Verification items for the finished model (mm, model axes). Face numbers are marked on the shaded views. A direction names the side the tool comes from. Coordinates: 2 decimals unless noted, no trailing zeros. Loops run counter-clockwise (first coordinate to the right, second up) from the corner with the lowest first, then second, coordinate; pieces in that order, holes last.
Q1. Access from +Z, -Z, +X, -X, +Y, -Y to the whole of each face (thin tool, end or side, straight path). Record for the marked faces 1, 2, 3 and 4.
Q2. Sectioned sample at D-D (z = 10). Enter the section's corners in (x, y).
Q3. Mould release check, pull along Z, two halves, no side actions. Record for the marked faces 5, 6 and 7: +Z half, -Z half, draft (parallel to the pull), parting line (faces both ways), or undercut.
Q4. Go/stop test with flat-tipped pins: P1, Ø6, axis at x = 2, y = 0, coming from the +Z side; P2, Ø4, axis at y = 2.5, z = 18.5, coming from the -X side; P3, Ø14, axis at y = -7, z = 25.5, coming from the +X side. Record where each tip stops, or that it passes through.
Q5. Sectioned sample at C-C (y = 0). Enter the section's corners in (x, z).
Q6. Sectioned sample at A-A (y = -30). Enter the section's corners in (x, z), then the cut area to 3 significant figures.
Q7. Sectioned sample at B-B (x = 10). Enter the section's corners in (y, z), then the cut area to 3 significant figures.
Q8. Material ranges on probe 1 along Y at (x, z) = (0, 28); probe 2 along Y at (x, z) = (-6.5, 3); probe 3 along X at (y, z) = (12, 28.75), recorded low to high.
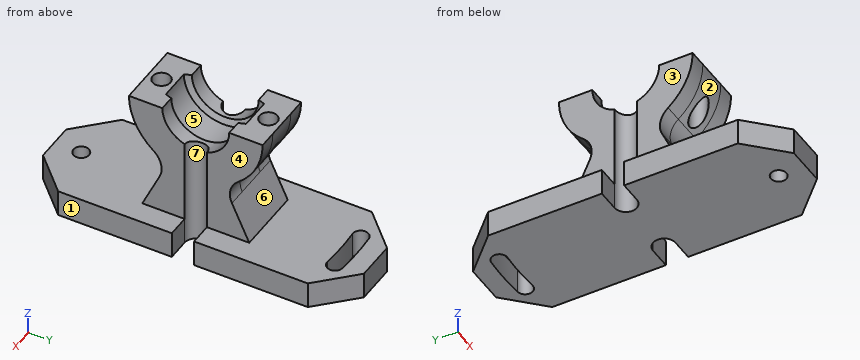
Autodesk Inventor part; units mm, degrees
ref_plane "YZ Plane" through (0, 0, 0) normal (1, 0, 0) x (0, 1, 0)
ref_plane "XZ Plane" through (0, 0, 0) normal (0, 1, 0) x (-1, 0, 0)
ref_plane "XY Plane" through (0, 0, 0) normal (0, 0, 1) x (1, 0, 0)
sketch "Sketch1" plane through (0, 0, 0) normal (1, 0, 0) x (0, 1, 0)
  line L0 (-36, 0) -> (36, 0)
  line L1 (36, 0) -> (36, 6)
  line L2 (36, 6) -> (-36, 6)
  line L3 (-36, 6) -> (-36, 0)
  circle A0 centre (0, 32) radius 9
  circle A1 centre (0, 32) radius 15
  line L4 (0, 32) -> (3.7715, 23.8284) construction
  line L5 (6.2859, 18.3806) -> (12, 6)
  line L6 (0, 32) -> (-3.7715, 23.8284) construction
  line L7 (-6.2859, 18.3806) -> (-12, 6)
  line L8 (15, 32) -> (9, 32)
  line L9 (-9, 32) -> (-15, 32)
  point P0 (0, 0)
  point P1 (0, 0)
  point P2 (12, 32)
  dimension "d3" = 18
  dimension "d4" = 32
  dimension "d5" = 6
  dimension "d6" = 72
  dimension "d7" = 6
  dimension "d44" = 12
  dimension "d45" = 12
extrude "Extrusion1" add sketch "Sketch1" along normal mid plane 7 contours L3 L2 L1 L0 | L7 A1 L5 L2 | A1 L9 A0 L8 picked at (12.871, 30.8714)
sketch "Sketch2" plane through (3.5, 0, 0) normal (1, 0, 0) x (0, 0, -1)
  line L0 (-6, 36) -> (-6, 12)
  line L1 (-6, 12) -> (-18.3806, 6.2859)
  arc A0 (-18.3806, 6.2859) -> (-32, 15) centre (-32, 0) ccw
  line L2 (-32, 15) -> (-32, 9)
  arc A1 (-32, -9) -> (-32, 9) centre (-32, 0) ccw
  line L3 (-32, -9) -> (-32, -15)
  arc A2 (-32, -15) -> (-18.3806, -6.2859) centre (-32, 0) ccw
  line L4 (-18.3806, -6.2859) -> (-6, -12)
  line L5 (-6, -12) -> (-6, -36)
  line L6 (-6, -36) -> (0, -36)
  line L7 (0, -36) -> (0, 36)
  line L8 (0, 36) -> (-6, 36)
  arc A3 (-32, -7.5) -> (-32, 7.5) centre (-32, 0) ccw
  line L9 (-32, 9) -> (-32, 7.5)
  line L10 (-32, -9) -> (-32, -15)
  line L11 (-32, -7.5) -> (-32, -9)
  point P0 (0, 0)
  dimension "d14" = 1.5
extrude "Extrusion2" add sketch "Sketch2" along normal blind 4
sketch "Sketch3" plane through (-3.5, 0, 0) normal (-1, 0, 0) x (0, 0, 1)
  arc A0 (18.3806, -6.2859) -> (32, -15) centre (32, 0) ccw
  line L0 (18.3806, -6.2859) -> (6, -12)
  line L1 (6, -12) -> (6, -36)
  line L2 (6, -36) -> (0, -36)
  line L3 (0, -36) -> (0, 36)
  line L4 (0, 36) -> (6, 36)
  line L5 (6, 36) -> (6, 12)
  line L6 (6, 12) -> (18.3806, 6.2859)
  arc A1 (32, 15) -> (18.3806, 6.2859) centre (32, 0) ccw
  line L7 (32, 15) -> (32, 7.5)
  arc A2 (32, 7.5) -> (32, -7.5) centre (32, 0) ccw
  line L8 (32, -7.5) -> (32, -15)
  point P0 (0, 0)
extrude "Extrusion3" add sketch "Sketch3" along normal blind 4
sketch "Sketch4" plane through (7.5, -36, 0) normal (0, 0, -1) x (-1, 0, 0)
  line L0 (15, 72) -> (15, 0)
  line L1 (0, 0) -> (0, 72)
  line L2 (15, 0) -> (20, 0)
  line L3 (20, 0) -> (20, 72)
  line L4 (20, 72) -> (15, 72)
  line L5 (15, 72) -> (15, 0)
  line L6 (0, 0) -> (-5, 0)
  line L7 (-5, 0) -> (-5, 72)
  line L8 (-5, 72) -> (0, 72)
  line L9 (0, 72) -> (0, 0)
  point P0 (7.5, 36)
  dimension "d17" = 25
extrude "Extrusion4" add sketch "Sketch4" against normal up to surface (6 mm away)
sketch "Sketch5" plane through (3.5, -9, 32) normal (0, 0, 1) x (1, 0, 0)
  line L0 (4, 9) -> (-11, 9)
  line L1 (-11, 9) -> (-31, 9) construction
  line L2 (-11, 1.5) -> (-11, 16.5)
  line L3 (-11, 11.5) -> (-31, 11.5)
  line L4 (-31, 6.5) -> (-11, 6.5)
  arc A0 (-11, 6.5) -> (-11, 11.5) centre (-11, 9) ccw
  arc A1 (-31, 11.5) -> (-31, 6.5) centre (-31, 9) ccw
  line L5 (4, 9) -> (24, 9) construction
  line L6 (4, 11.5) -> (24, 11.5)
  line L7 (24, 6.5) -> (4, 6.5)
  arc A2 (4, 11.5) -> (4, 6.5) centre (4, 9) ccw
  arc A3 (24, 6.5) -> (24, 11.5) centre (24, 9) ccw
  point P0 (-3.5, 9)
  point P1 (-3.5, 9)
  point P2 (-21, 9)
  point P3 (14, 9)
  dimension "d20" = 15
  dimension "d52" = 20
  dimension "d53" = 20
  dimension "d54" = 5
sketch "Sketch8" plane through (3.5, -9, 32) normal (0, 0, 1) x (1, 0, 0)
  line L0 (-11, -6) -> (4, -6)
  line L1 (4, 1.5) -> (4, -6)
  line L2 (0, 1.5) -> (4, 1.5)
  line L3 (0, 1.5) -> (0, 0)
  line L4 (-7, 0) -> (0, 0)
  line L5 (-7, 0) -> (-7, 1.5)
  line L6 (-7, 1.5) -> (-11, 1.5)
  line L7 (-11, -6) -> (-11, 1.5)
  line L8 (-7, 18) -> (0, 18)
  line L9 (0, 18) -> (0, 16.5)
  line L10 (0, 16.5) -> (4, 16.5)
  line L11 (4, 24) -> (4, 16.5)
  line L12 (-11, 24) -> (4, 24)
  line L13 (-11, 16.5) -> (-11, 24)
  line L14 (-7, 16.5) -> (-11, 16.5)
  line L15 (-7, 16.5) -> (-7, 18)
  line L16 (-7, 0) -> (0, 0)
  line L17 (-3.5, 0) -> (-3.5, -6)
  line L18 (-7, 18) -> (0, 18)
  line L19 (-3.5, 18) -> (-3.5, 24)
  line L20 (-11, 24) -> (4, 24)
  line L21 (-16, -27) -> (9, -27)
  line L22 (-16, 45) -> (9, 45)
  point P0 (-3.5, 9)
  point P1 (-3.5, -3)
  point P2 (-3.5, 21)
hole "Hole2" at (0, -12, 32) at (0, 12, 32) direction (0, 0, -1) diameter 4 depth 16
sketch "Sketch6" plane through (3.5, -9, 32) normal (0, 0, 1) x (1, 0, 0)
  line L0 (-11, -6) -> (4, -6)
  line L1 (4, 1.5) -> (4, -6)
  line L2 (0, 1.5) -> (4, 1.5) construction
  line L3 (0, 1.5) -> (0, 0)
  line L4 (-7, 0) -> (0, 0)
  line L5 (-7, 0) -> (-7, 1.5)
  line L6 (-7, 1.5) -> (-11, 1.5) construction
  line L7 (-11, -6) -> (-11, 1.5)
  line L8 (9, 45) -> (9, -27)
  line L9 (9, 9) -> (-16, 9)
  line L10 (-16, -27) -> (-16, 45)
  line L11 (-7, 18) -> (0, 18)
  line L12 (0, 18) -> (0, 16.5)
  line L13 (0, 16.5) -> (4, 16.5)
  line L14 (4, 24) -> (4, 16.5)
  line L15 (-11, 24) -> (4, 24)
  line L16 (-11, 16.5) -> (-11, 24)
  line L17 (-7, 16.5) -> (-11, 16.5)
  line L18 (-7, 16.5) -> (-7, 18)
  line L19 (0, 1.5) -> (4, 1.5)
  line L20 (0, 16.5) -> (0, 1.5)
  line L21 (-7, 1.5) -> (-7, 16.5)
  line L22 (-7, 1.5) -> (-11, 1.5)
  arc A0 (0, 0) -> (0, 18) centre (-23.3238, 9) ccw
  arc A1 (-7, 18) -> (-7, 0) centre (16.3238, 9) ccw
  point P0 (-3.5, 9)
  point P1 (-7, 9)
  point P2 (-8.6762, 9)
  point P3 (1.6762, 9)
  point P4 (0, 9)
  dimension "d30" = 25
  dimension "d31" = 25
revolve "Revolution1" cut sketch "Sketch6" angle 360 about axis through (12.5, 0, 32) along (-1, 0, 0) contours A1 L9 L21 L22 | L22 L5 A1 | A0 L3 L19 | L19 L20 L9 A0
fillet "Fillet1" radius 5 2 edges at (0, 6.2859, 18.3806) (0, -6.2859, 18.3806)
sketch "Sketch10" plane through (-12.5, 36, 6) normal (0, 0, 1) x (1, 0, 0)
  line L0 (12.5, -66) -> (12.5, -6)
  line L1 (0, 0) -> (25, 0)
  circle A0 centre (12.5, -66) radius 1.75
  arc A1 (17.5, -6.2087) -> (7.5, -6.2087) centre (12.5, -66) ccw construction
  arc A2 (17.6458, -4.4648) -> (7.3542, -4.4648) centre (12.5, -66) ccw
  arc A3 (17.3542, -7.9526) -> (7.6458, -7.9526) centre (12.5, -66) ccw
  arc A4 (17.3542, -7.9526) -> (17.6458, -4.4648) centre (17.5, -6.2087) ccw
  arc A5 (7.3542, -4.4648) -> (7.6458, -7.9526) centre (7.5, -6.2087) ccw
  point P0 (12.5, -36)
  point P1 (12.5, -36)
  dimension "d46" = 60
  dimension "d47" = 3.5
  dimension "d48" = 3.5
  dimension "d49" = 5
extrude "Extrusion5" cut sketch "Sketch10" against normal through all
extrude "Extrusion6" cut sketch "Sketch5" against normal up to surface (32 mm away)
chamfer "Chamfer1" distance 8 angle 45 4 edges at (12.5, 36, 3) (-12.5, 36, 3) (12.5, -36, 3) (-12.5, -36, 3)
equation "\"d3\" = LENS_D"
equation "\"d10\" = LENS_L"
equation "\"d30\" = LENS_R"
equation "\"d31\" = LENS_R"
equation "\"LENS_D\" = 18"
equation "\"LENS_L\" = 7"
equation "\"LENS_R\" = 25"
properties part number "LensHolder"
Geometry check:
1. face 1: +Z, -Z, +X, +Y, -Y
1. face 2: +X, -X, -Y
1. face 3: +Z, -X, +Y, -Y
1. face 4: +Z, +X, +Y, -Y
2. outline: (-7.5, -10.15) - (7.5, -10.15) - (7.5, -2.5) arc R2.5 cw to (7.5, 2.5) - (7.5, 10.15) - (-7.5, 10.15) - (-7.5, 2.5) arc R2.5 cw to (-7.5, -2.5) - close
3. face 5: +Z half
3. face 6: undercut
3. face 7: draft
4. P1: stops at z = 24.83
4. P2: stops at x = -7.5
4. P3: stops at x = 7.5
5. outline: (-5, 0) - (5, 0) - (5, 24.5) - (4.02, 24.5) arc R25 cw to (3.5, 23) - (-3.5, 23) arc R25 cw to (-4.02, 24.5) - (-5, 24.5) - close
6. outline: (-10.5, 0) - (-1.75, 0) - (-1.75, 6) - (-10.5, 6) - close; (1.75, 0) - (10.5, 0) - (10.5, 6) - (1.75, 6) - close
6. area: 105 mm2
7. outline: (-30.5, 0) - (-2.5, 0) - (-2.5, 6) - (-30.5, 6) - close; (2.5, 0) - (30.5, 0) - (30.5, 6) - (2.5, 6) - close
7. area: 336 mm2
8. probe 1: y = -14.46 to -14, -10 to -8.06, 8.06 to 10, 14 to 14.46
8. probe 2: y = -34 to -2.29, 2.29 to 28.89, 30.69 to 34
8. probe 3: x = -7.5 to -2, 2 to 7.5
